Autodesk Inventor part; units mm, degrees
ref_plane "YZ Plane" through (0, 0, 0) normal (1, 0, 0) x (0, 1, 0)
ref_plane "XZ Plane" through (0, 0, 0) normal (0, 1, 0) x (-1, 0, 0)
ref_plane "XY Plane" through (0, 0, 0) normal (0, 0, 1) x (1, 0, 0)
sketch "スケッチ1" plane through (0, 0, 0) normal (0, 1, 0) x (-1, 0, 0)
  line L0 (-6.2, 0) -> (-10.5, 0)
  line L1 (-10.5, 0) -> (-10.5, 3.5)
  line L2 (-10.5, 3.5) -> (-6.85, 3.5)
  line L3 (-6.85, 3.5) -> (-6.85, 2.7)
  line L4 (-6.85, 2.7) -> (-6.8, 2.7)
  line L5 (-6.8, 3.4) -> (-6.8, 2.7)
  line L6 (-6, 0.2) -> (-6, 0.1)
  line L7 (-5.9, 0) -> (-4.1, 0)
  line L8 (-4, 0.1) -> (-4, 3.4)
  line L9 (-4.1, 3.5) -> (-6.7, 3.5)
  line L10 (0, -0.729) -> (0, 4.229)
  line L11 (-6, 0.2) -> (-6.2, 0)
  arc A0 (-6.7, 3.5) -> (-6.8, 3.4) centre (-6.7, 3.4) ccw
  arc A1 (-4, 3.4) -> (-4.1, 3.5) centre (-4.1, 3.4) ccw
  arc A2 (-4.1, 0) -> (-4, 0.1) centre (-4.1, 0.1) ccw
  arc A3 (-6, 0.1) -> (-5.9, 0) centre (-5.9, 0.1) ccw
  line L12 (2.1, 0) -> (-12.6, 0)
  line L13 (-10.5, 1.75) -> (-4, 1.75) construction
  line L14 (-6.85, 0) -> (-6.85, 0.8)
  line L15 (-6.85, 0.8) -> (-6.8, 0.8)
  line L16 (-6.8, 0.1) -> (-6.8, 0.8)
  line L17 (-6, 3.3) -> (-6, 3.4)
  line L18 (-6, 3.3) -> (-6.2, 3.5)
  arc A4 (-6.8, 0.1) -> (-6.7, 0) centre (-6.7, 0.1) ccw
  arc A5 (-5.9, 3.5) -> (-6, 3.4) centre (-5.9, 3.4) ccw
  line L19 (-6.2, 0) -> (-5.9, 0)
  line L20 (-6.7, 3.5) -> (-6.85, 3.5)
  point P0 (0, 0)
  point P1 (-6.8, 3.5)
  point P2 (-6, 0)
  point P3 (-4, 0)
  point P4 (-4, 3.5)
  point P5 (-5.9, 3.5)
  point P6 (-6.7, 0)
  dimension "d0" = 8
  dimension "d1" = 21
  dimension "d2" = 0.8
  dimension "d3" = 0.1
  dimension "d4" = 13.7
  dimension "d5" = 13.6
  dimension "d6" = 0.2
  dimension "d7" = 0.2
  dimension "d8" = 12
  dimension "d9" = 3.5
revolve "回転1" add sketch "スケッチ1" angle 360 about axis through (0, 0, -10) along (0, 0, 1) contours L0 A4 L16 L15 L14 L1 L2 L3 L4 L5 A0 L9 L18 L17 A5 A1 L8 A2 L7 A3 L6 L11 | L11 L6 A3 L12 | L20 A0 L5 L4 L3
sketch "スケッチ2" plane through (0, 0, 3.5) normal (0, 0, 1) x (1, 0, 0)
  line L0 (-14.7, 0) -> (14.7, 0)
  point P0 (0, 0)
  point P1 (-8.5, 0)
  dimension "d12" = 8.5
hole "穴1" at (-8.5, 0, 3.5) direction (0, 0, -1) diameter 2.1129 end through all
pattern_circular "円形状パターン1" count 8 over 360 about axis through (0, 0, -10) along (0, 0, 1) of "穴1"
chamfer "面取り1" distance 0.2 angle 45 2 edges at (-10.5, 0, 3.5) (-10.5, 0, 0)
properties part number "FreeHorn" material "アルミニウム 2014-T4"
Design review of the part built by this model. Coordinates are the model's own, in mm. Round coordinates to 2 decimals unless told otherwise and drop trailing zeros. One line per question, with ' | ' between items.
1. Clearance check with flat-ended pins moving along their axes: P1, Ø1.3, axis at x = -6.01, y = 6.01, coming from the -Z side; P2, Ø2, axis at y = -3, z = 2, coming from the -X side; P3, Ø1, axis at y = -2.5, z = 3, coming from the +X side. State where each tip first meets the part, or that it passes through.
Results are:
P1: passes through | P2: stops at x = -10.31 | P3: stops at x = 10.31
2. We need section A-A, the plane z = 0.55. State how many separate pieces and enclosed holes the cut face has, and give its area (3 significant figures).
Results are:
separate pieces: 2 | enclosed holes: 10 | area: 266 mm²
3. Draft analysis for pull direction Y (two halves, no side actions). For faces 1 (the face through (-0.23, -7.47, 1.73)), 2 (the face through (10, 3.2, 1.8)), 3 (the face through (-0.1, -4.4, 0)), state which applies: released by +Y, released by -Y, zero draft, split by the parting line, or undercut.
Results are:
face 1: undercut | face 2: split by the parting line | face 3: zero draft
4. For L1, parallel to Y at x = 0, z = 1.5; L2, parallel to Y at x = -0.5, z = 2.2, list the stretches that pass through material, from the lowest coordinate up. Write a range as [from, to].
Results are:
L1: y = [-10.5, -9.56], [-7.44, -4], [4, 7.44], [9.56, 10.5] | L2: y = [-10.49, -9.43], [-7.57, -3.97], [3.97, 7.57], [9.43, 10.49]
